Geometry: final body of the model. Coordinates: model frame, mm. A direction names the side the tool comes from. Give positions to 0.01 mm unless a question says otherwise; leave off trailing zeros. Loops run counter-clockwise (first coordinate to the right, second up) from the corner with the lowest first, then second, coordinate; pieces in that order, holes last.
from build123d import *

# Parameters (mm, degrees)
EXTRUDE_1_DEPTH     = 200
SKETCH_2_W          = 1.5
SKETCH_2_H          = 18.5
CUT_EXTRUDE_1_DEPTH = 20
CUT_EXTRUDE_2_REACH = 203.99
SKETCH_3_R          = 1.75


with BuildPart() as part:
    # Эскиз1 → Бобышка-Вытянуть1 (new body)
    with BuildSketch(Plane(origin=(0, 0, 0), x_dir=(1, 0, 0), z_dir=(0, 1, 0))):
        Polygon((0, 0), (0, 20), (1.5, 20), (1.5, 1.5), (20, 1.5), (20, 0), align=None)
    extrude(amount=EXTRUDE_1_DEPTH)

    # Эскиз2 → Вырез-Вытянуть1 (cut)
    with BuildSketch(Plane(origin=(0, 200, 0), x_dir=(1, 0, 0), z_dir=(0, 1, 0))):
        with Locations((0.75, 10.75)):
            Rectangle(SKETCH_2_W, SKETCH_2_H)
    cut_extrude_1 = extrude(amount=-CUT_EXTRUDE_1_DEPTH, mode=Mode.SUBTRACT)

    # Эскиз3 → Вырез-Вытянуть2 (cut, up to next)
    with BuildSketch(Plane.XY, mode=Mode.PRIVATE) as cut_extrude_2_sk1:
        with Locations((10, 190)):
            Circle(SKETCH_3_R)
    cut_extrude_2_tool1 = extrude(cut_extrude_2_sk1.sketch, amount=-CUT_EXTRUDE_2_REACH, mode=Mode.PRIVATE) & part.part
    cut_extrude_2 = cut_extrude_2_tool1.solids().sort_by_distance((10, 190, 0))[0]
    add(cut_extrude_2, mode=Mode.SUBTRACT)

    # Зеркальное отражение1: Вырез-Вытянуть1, Вырез-Вытянуть2 across plane
    add(cut_extrude_1.mirror(Plane(origin=(0, 100, 0), x_dir=(0, 0, 1), z_dir=(0, -1, 0))), mode=Mode.SUBTRACT)
    add(cut_extrude_2.mirror(Plane(origin=(0, 100, 0), x_dir=(0, 0, 1), z_dir=(0, -1, 0))), mode=Mode.SUBTRACT)


solid = part.part
Item 1: Section query B-B on x = 10. Return loops of the section in (y, z).
Values follow:
outline: (0, -1.5) - (8.25, -1.5) - (8.25, 0) - (0, 0) - close; (11.75, -1.5) - (188.25, -1.5) - (188.25, 0) - (11.75, 0) - close; (191.75, -1.5) - (200, -1.5) - (200, 0) - (191.75, 0) - close
Item 2: Pin query (flat end, axial travel): pin 1 (1.6 mm diameter, centred on x = 0.5, z = -11, fed in from -Y); pin 2 (5.5 mm diameter, centred on y = 82, z = -14, fed in from +X); pin 3 (1.5 mm diameter, centred on x = 9, y = 152, fed in from -Z). Return the tip coordinate at first contact, or that it passes through.
Values follow:
pin 1: stops at y = 20
pin 2: stops at x = 1.5
pin 3: stops at z = -1.5
Item 3: Set-up query: faces 1 (the face through (1.5, 99, -11)), 2 (the face through (10.81, 188.45, -0.74)). Return all of +Z, -Z, +X, -X, +Y, -Y with unobstructed straight access to the full face (end or side cutting, diameter ignored); none if empty.
Values follow:
face 1: -Z, +X, +Y, -Y
face 2: +Z, -Z
Item 4: Section query D-D on y = 137.5. Return loops of the section in (x, z), plus the area to 4 significant figures.
Values follow:
outline: (0, -20) - (1.5, -20) - (1.5, -1.5) - (20, -1.5) - (20, 0) - (0, 0) - close
area: 57.75 mm2
Item 5: Ray query, probe 1 along Y at (x, z) = (10, -0.7); probe 2 along X at (y, z) = (10, -0.9); probe 3 along X at (y, z) = (112, -15.75). Return the intervals inside material, ascending.
Values follow:
probe 1: y = 0 to 8.25, 11.75 to 188.25, 191.75 to 200
probe 2: x = 0 to 8.25, 11.75 to 20
probe 3: x = 0 to 1.5
Item 6: Draft query along Y for faces 3 (the face through (10, 99, -1.5)), 4 (the face through (10.9, 8.5, -0.7)). Return one class per face: +Y half, -Y half, draft (parallel to the pull), parting line (faces both ways), or undercut.
Values follow:
face 3: draft
face 4: undercut
Item 7: Section query A-A on y = 190. Return loops of the section in (x, z).
Values follow:
outline: (0, -1.5) - (8.25, -1.5) - (8.25, 0) - (0, 0) - close; (11.75, -1.5) - (20, -1.5) - (20, 0) - (11.75, 0) - close
Item 8: Section query C-C on z = -18.25. Return loops of the section in (x, y), plus the area to 3 significant figures.
Values follow:
outline: (0, 20) - (1.5, 20) - (1.5, 180) - (0, 180) - close
area: 240 mm2
